Could you check a few things on this drawing? It's one solid part, dimensions in mm from its lowest x, y, z. A direction names the side the tool comes from. Coordinates: 2 decimals unless noted, no trailing zeros. Write each loop counter-clockwise with the first axis right and the second up, starting at its lowest first coordinate (ties: lowest second). Pieces come first, ordered by that corner, then holes.
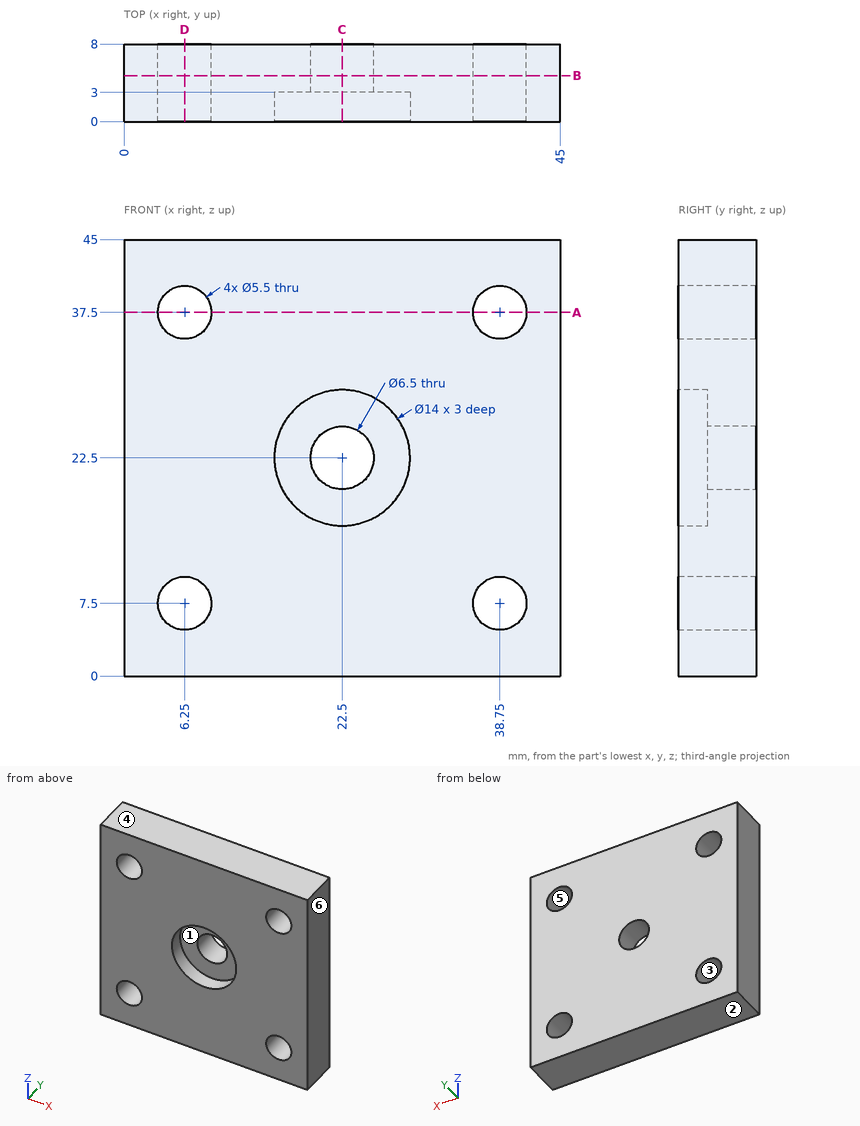
1) Imagine slicing it at C-C on x = 22.5. Please give me the cut outline in (y, z), then the cut area to 4 significant figures.
Values follow:
outline: (0, 0) - (8, 0) - (8, 19.25) - (3, 19.25) - (3, 15.5) - (0, 15.5) - close; (0, 29.5) - (3, 29.5) - (3, 25.75) - (8, 25.75) - (8, 45) - (0, 45) - close
area: 285.5 mm2
2) I need wall thicknesses on probe 1 along X at (y, z) = (6, 7.5); probe 2 along X at (y, z) = (4.5, 39.5); probe 3 along X at (y, z) = (6.95, 22.5). Which ranges of each line are inside material? Lowest first, please.
Values follow:
probe 1: x = 0 to 3.5, 9 to 36, 41.5 to 45
probe 2: x = 0 to 4.36, 8.14 to 36.86, 40.64 to 45
probe 3: x = 0 to 19.25, 25.75 to 45
3) Imagine slicing it at A-A on z = 37.5. Please give me the cut outline in (x, y).
Values follow:
outline: (0, 0) - (3.5, 0) - (3.5, 8) - (0, 8) - close; (9, 0) - (36, 0) - (36, 8) - (9, 8) - close; (41.5, 0) - (45, 0) - (45, 8) - (41.5, 8) - close
4) We'd pull the mould along Z, two halves only. Please class the marked faces 3, 4, 5 and 6: pulls with the +Z half, pulls with the -Z half, needs draft (parallel to the pull), parting line crosses it, or undercut.
Values follow:
face 3: undercut
face 4: pulls with the +Z half
face 5: undercut
face 6: needs draft
5) Imagine slicing it at B-B on y = 4.75. Please give me the cut outline in (x, z), then the cut area to 3 significant figures.
Values follow:
outline: (0, 0) - (45, 0) - (45, 45) - (0, 45) - close; hole circle Ø5.5 at (6.25, 7.5); hole circle Ø5.5 at (6.25, 37.5); hole circle Ø6.5 at (22.5, 22.5); hole circle Ø5.5 at (38.75, 7.5); hole circle Ø5.5 at (38.75, 37.5)
area: 1,900 mm2
6) Imagine slicing it at D-D on x = 6.25. Please give me the cut outline in (y, z), then the cut area to 3 significant figures.
Values follow:
outline: (0, 0) - (8, 0) - (8, 4.75) - (0, 4.75) - close; (0, 10.25) - (8, 10.25) - (8, 34.75) - (0, 34.75) - close; (0, 40.25) - (8, 40.25) - (8, 45) - (0, 45) - close
area: 272 mm2
7) Will these pins go through, and if not, where does the flat tip stop? pin 1 (12.5 mm diameter, centred on x = 22.5, z = 22.5, fed in from -Y); pin 2 (5 mm diameter, centred on x = 6.25, z = 7.5, fed in from +Y).
Values follow:
pin 1: stops at y = 3
pin 2: passes through
8) On a 3-axis mill with a long thin cutter (end or side, diameter ignored), from which of +Z, -Z, +X, -X, +Y, -Y can I reach the whole of each face in a straight line? I mean the marked faces 1 and 2. Say none if no direction works.
Values follow:
face 1: -Y
face 2: -Z, +X, -X, +Y, -Y
